Check sheet for the drawn part. Datum: minimum x, y, z corner. Units: mm. A direction names the side the tool comes from. Coordinates: 2 decimals unless noted, no trailing zeros. Write each loop counter-clockwise with the first axis right and the second up, starting at its lowest first coordinate (ties: lowest second). Pieces come first, ordered by that corner, then holes. Notation, with made-up numbers: M 73,84 L 85,84 A31 cw 85,117 Z; hole C 75,24.25 d8. An arc over 180 degrees is marked long. Answer as CSV lines item,"result".
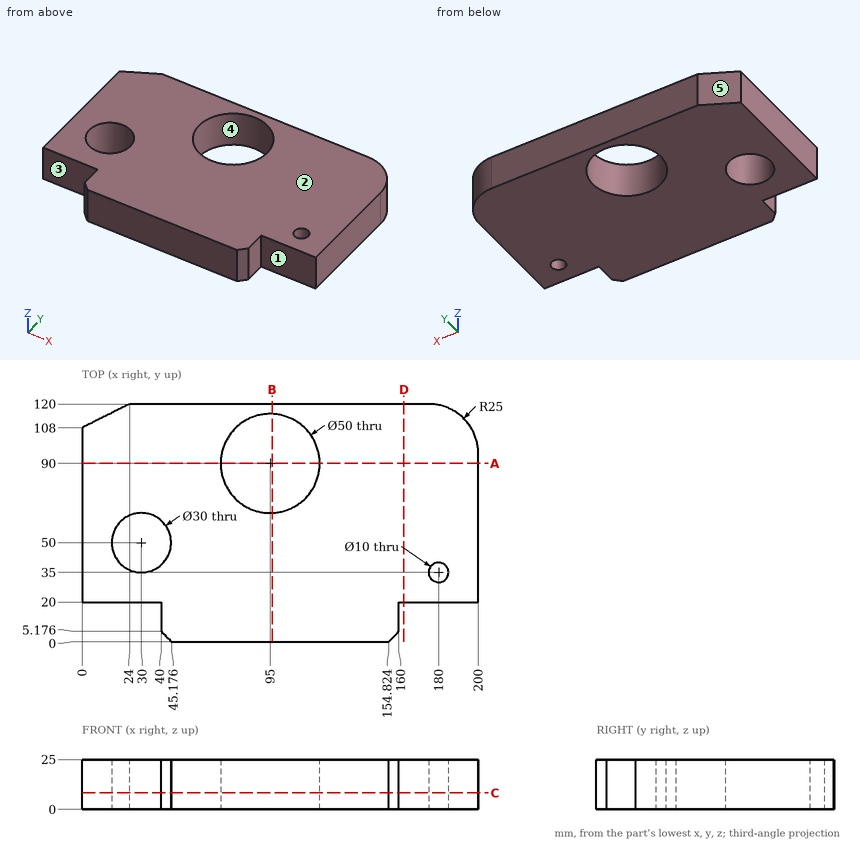
1) Mould release check, pull along X, two halves, no side actions. Record for the marked faces 3, 4 and 5: pulls with the +X half, pulls with the -X half, needs draft (parallel to the pull), parting line crosses it, or undercut.
Answer key:
face 3,"needs draft"
face 4,"undercut"
face 5,"pulls with the -X half"
2) Tool access check on the marked faces 1 and 2. Record the directions out of +Z, -Z, +X, -X, +Y, -Y that give a thin tool (end or side, any length) a straight path to the whole face; none if there is none.
Answer key:
face 1,"+Z, -Z, +X, -Y"
face 2,"+Z, +X, -X, +Y, -Y"
3) Thickness scan on line 1 along Y through (x, z) = (31, 24.25); line 2 along Y through (x, z) = (95, 5.75); line 3 along X through (y, z) = (38, 3.5). Record the ranges inside material, lowest first.
Answer key:
line 1,"y = 20 to 35.03, 64.97 to 120"
line 2,"y = 0 to 65, 115 to 120"
line 3,"x = 0 to 21, 39 to 176, 184 to 200"
4) Section check C-C, the plane z = 8.25. Record the boundary of the cut face in (x, y).
Answer key:
outline,"M 0,20 L 40,20 L 40,5.18 L 45.18,0 L 154.82,0 L 160,5.18 L 160,20 L 200,20 L 200,95 A25 ccw 175,120 L 24,120 L 0,108 Z; hole C 30,50 d30; hole C 95,90 d50; hole C 180,35 d10"
5) Depth check by flat-ended pin: P1, Ø12, axis at y = 11, z = 13.5, coming from the -X side; P2, Ø24, axis at x = 30, y = 50, coming from the -Z side; P3, Ø12.5, axis at x = 26, z = 10, coming from the -Y side. Enter the tip coordinate at first touch or a pass-through.
Answer key:
P1,"stops at x = 40"
P2,"passes through"
P3,"stops at y = 20"
6) Section check A-A, the plane y = 90. Record the boundary of the cut face in (x, z), plus the area to 3 significant figures.
Answer key:
outline,"M 0,0 L 70,0 L 70,25 L 0,25 Z; M 120,0 L 200,0 L 200,25 L 120,25 Z"
area,"3,750 mm2"
7) Section check B-B, the plane x = 96. Record the boundary of the cut face in (y, z), plus the area to 3 significant figures.
Answer key:
outline,"M 0,0 L 65.02,0 L 65.02,25 L 0,25 Z; M 114.98,0 L 120,0 L 120,25 L 114.98,25 Z"
area,"1,750 mm2"
8) Section check D-D, the plane x = 162.5. Record the boundary of the cut face in (y, z), plus the area to 3 significant figures.
Answer key:
outline,"M 20,0 L 120,0 L 120,25 L 20,25 Z"
area,"2,500 mm2"
